Verification items for the finished model (mm, model axes). A direction names the side the tool comes from. Round coordinates to 2 decimals unless told otherwise and drop trailing zeros. Write each loop counter-clockwise with the first axis right and the second up, starting at its lowest first coordinate (ties: lowest second). Pieces come first, ordered by that corner, then holes. Notation, with made-up numbers: (-1.75, -39) -> (57.25, -39) arc R23 cw to (57.25, -15) -> close; hole circle Ø11 at (-24, 6). An arc over 180 degrees is marked (long way). Use CSV: the item, a comma, the result in double quotes.
```python
from build123d import *
from build123d.topology import SkipClean

# Parameters (mm, degrees)
BOSS_EXTRUDE2_DEPTH       = 12.065
BOSS_EXTRUDE3_START       = -15.875
BOSS_EXTRUDE3_OUTLINE_R   = 38.1
BOSS_EXTRUDE3_OUTLINE_R_2 = 25.4
BOSS_EXTRUDE3_DEPTH       = 31.75
SKETCH3_R                 = 9.525
BOSS_EXTRUDE4_DEPTH       = 25.4
SKETCH5_R                 = 4.76
CUT_EXTRUDE1_DEPTH        = 32.4


# Read off the part's stored shape, not the designer's step: Boss-Extrude3
with BuildPart() as part:
    # Sketch1 → Boss-Extrude2 (new, symmetric)
    with SkipClean():  # the faces are left unmerged after this step: merging them gives an invalid solid
        with BuildSketch(Plane(origin=(0, 0, 0), x_dir=(0, 0, -1), z_dir=(1, 0, 0))):
            with BuildLine():
                ThreePointArc((-43.204432116, 19.05), (-114.3, 0), (-43.204432116, -19.05))
                Line((-43.204432116, -19.05), (-59.399479175, -19.05))
                ThreePointArc((-59.399479175, -19.05), (-101.6, 0), (-59.399479175, 19.05))
                Line((-59.399479175, 19.05), (-43.204432116, 19.05))
            make_face()
            with BuildLine():
                Line((-59.399479175, -19.05), (-43.204432116, -19.05))
                ThreePointArc((-43.204432116, -19.05), (-39.398226018, -9.861005618), (-38.1, 0))
                ThreePointArc((-38.1, 0), (-39.398226018, 9.861005618), (-43.204432116, 19.05))
                Line((-43.204432116, 19.05), (-59.399479175, 19.05))
                ThreePointArc((-59.399479175, 19.05), (-53.049479175, 10.450520825), (-50.8, 0))
                ThreePointArc((-50.8, 0), (-53.049479175, -10.450520825), (-59.399479175, -19.05))
            make_face()
            with BuildLine():
                Line((-43.204432116, -19.05), (29.107139607, -19.05))
                ThreePointArc((29.107139607, -19.05), (25.4, 0), (29.107139607, 19.05))
                Line((29.107139607, 19.05), (-43.204432116, 19.05))
                ThreePointArc((-43.204432116, 19.05), (-39.398226018, 9.861005618), (-38.1, 0))
                ThreePointArc((-38.1, 0), (-39.398226018, -9.861005618), (-43.204432116, -19.05))
            make_face()
            with BuildLine():
                Line((29.107139607, -19.05), (43.204432116, -19.05))
                ThreePointArc((43.204432116, -19.05), (38.1, 0), (43.204432116, 19.05))
                Line((43.204432116, 19.05), (29.107139607, 19.05))
                ThreePointArc((29.107139607, 19.05), (25.4, 0), (29.107139607, -19.05))
            make_face()
            with BuildLine():
                Line((29.107139607, 19.05), (43.204432116, 19.05))
                ThreePointArc((43.204432116, 19.05), (57.15, 32.995567884), (76.2, 38.1))
                Line((76.2, 38.1), (76.2, 50.8))
                ThreePointArc((76.2, 50.8), (47.801936686, 42.121134838), (29.107139607, 19.05))
            make_face()
            with BuildLine():
                ThreePointArc((76.2, -38.1), (57.15, -32.995567884), (43.204432116, -19.05))
                Line((43.204432116, -19.05), (29.107139607, -19.05))
                ThreePointArc((29.107139607, -19.05), (47.801936686, -42.121134838), (76.2, -50.8))
                Line((76.2, -50.8), (76.2, -38.1))
            make_face()
        extrude(amount=BOSS_EXTRUDE2_DEPTH, both=True)

    # Boss-Extrude3 outline → Boss-Extrude3 (add)
    with SkipClean():  # the faces are left unmerged after this step: merging them gives an invalid solid
        with BuildSketch(Plane(origin=(0, 0, 0), x_dir=(0, 0, -1), z_dir=(1, 0, 0)).offset(BOSS_EXTRUDE3_START)):
            with Locations((-76.2, 0)):
                Circle(BOSS_EXTRUDE3_OUTLINE_R)
            with Locations((-76.2, 0)):
                Circle(BOSS_EXTRUDE3_OUTLINE_R_2, mode=Mode.SUBTRACT)
        extrude(amount=BOSS_EXTRUDE3_DEPTH)
    add(part.part.scale(1), mode=Mode.REPLACE)  # the faces are merged on a copy

    # Sketch3 → Boss-Extrude4 (add)
    with BuildSketch(Plane(origin=(0, 0, -76.2), x_dir=(-1, 0, 0), z_dir=(0, 0, -1))):
        with Locations((0, -50.8)):
            Circle(SKETCH3_R)
    boss_extrude4 = extrude(amount=-BOSS_EXTRUDE4_DEPTH)

    # Sketch5 → Cut-Extrude1 (cut)
    with BuildSketch(Plane(origin=(0, 0, -76.2), x_dir=(-1, 0, 0), z_dir=(0, 0, -1))):
        with Locations((0, -50.8)):
            Circle(SKETCH5_R)
    cut_extrude1 = extrude(amount=-CUT_EXTRUDE1_DEPTH, mode=Mode.SUBTRACT)

    # Mirror2: Boss-Extrude4, Cut-Extrude1 across plane
    add(boss_extrude4.mirror(Plane.ZX))
    add(cut_extrude1.mirror(Plane.ZX), mode=Mode.SUBTRACT)


solid = part.part
```
Q1. Section check D-D (y = 22). Record the cut outline in (x, z) (3 decimals).
Filled in:
outline,"(-15.875, 45.094) -> (15.875, 45.094) -> (15.875, 63.505) -> (-15.875, 63.505) -> close; (-15.875, 88.895) -> (15.875, 88.895) -> (15.875, 107.306) -> (-15.875, 107.306) -> close; (-12.065, -45.094) -> (12.065, -45.094) -> (12.065, -30.411) -> (-12.065, -30.411) -> close"
Q2. Mould release check, pull along Z, two halves, no side actions. Record for faces 4 (the flat face through (0, -44, -76.2)), 5 (the flat face through (-15.875, -25, 68)), 6 (the cylindrical face through (0.169, -37.742, -42.197)): released by +Z, released by -Z, zero draft, split by the parting line, or undercut.
Filled in:
face 4,"released by -Z"
face 5,"zero draft"
face 6,"undercut"
Q3. Section check B-B (z = 86.5). Record the cut outline in (x, y) (3 decimals), plus the area to 3 significant figures.
Filled in:
outline,"(-15.875, -36.681) -> (15.875, -36.681) -> (15.875, -23.218) -> (-15.875, -23.218) -> close; (-15.875, 23.218) -> (15.875, 23.218) -> (15.875, 36.681) -> (-15.875, 36.681) -> close"
area,"855 mm²"
Q4. Access from +Z, -Z, +X, -X, +Y, -Y to the whole of each face (thin tool, end or side, straight path). Record for faces 1 (the flat face through (0, -56, -50.8)), 2 (the flat face through (0, 19.05, 7)), 3 (the flat face through (0, 56, -50.8)).
Filled in:
face 1,"+Z, +X, -X, -Y"
face 2,"+X, -X, +Y"
face 3,"+Z, +X, -X, +Y"
Q5. Section check A-A (x = 0). Record the cut outline in (y, z) (3 decimals), plus the area to 3 significant figures.
Filled in:
outline,"(-60.325, -76.2) -> (-55.56, -76.2) -> (-55.56, -50.8) -> (-60.325, -50.8) -> close; (-46.04, -76.2) -> (-38.1, -76.2) arc R38.1 cw to (38.1, -76.2) -> (46.04, -76.2) -> (46.04, -50.8) -> (43.994, -50.8) arc R50.8 ccw to (19.05, -29.107) -> (19.05, 43.204) arc R38.1 ccw (long way) to (-19.05, 43.204) -> (-19.05, -29.107) arc R50.8 ccw to (-43.994, -50.8) -> (-46.04, -50.8) -> close; (55.56, -76.2) -> (60.325, -76.2) -> (60.325, -50.8) -> (55.56, -50.8) -> close; hole circle Ø50.8 at (0, 76.2)"
area,"6,950 mm²"
Q6. Section check C-C (y = -4.5). Record the cut outline in (x, z) (3 decimals), plus the area to 3 significant figures.
Filled in:
outline,"(-15.875, 38.367) -> (-12.065, 38.367) -> (-12.065, -38.367) -> (12.065, -38.367) -> (12.065, 38.367) -> (15.875, 38.367) -> (15.875, 51.202) -> (-15.875, 51.202) -> close; (-15.875, 101.198) -> (15.875, 101.198) -> (15.875, 114.033) -> (-15.875, 114.033) -> close"
area,"2,670 mm²"
Q7. Material ranges on L1, parallel to Y at x = 0, z = -60.25 (3 decimals); L2, parallel to Y at x = 0, z = -68 (3 decimals); L3, parallel to Y at x = -13.65, z = 76.2, recorded low to high.
Filled in:
L1,"-60.325 to -55.56, -46.04 to -34.601, 34.601 to 46.04, 55.56 to 60.325"
L2,"-60.325 to -55.56, -46.04 to -37.207, 37.207 to 46.04, 55.56 to 60.325"
L3,"-38.1 to -25.4, 25.4 to 38.1"
Q8. Go/stop test with flat-tipped pins: P1, Ø8, axis at x = -4.5, y = -52, coming from the +Z side; P2, Ø12, axis at x = 0, z = -4, coming from the +Y side; P3, Ø8, axis at y = -22.5, z = -36, coming from the +X side (3 decimals). Record where each tip stops, or that it passes through.
Filled in:
P1,"z = -50.8"
P2,"y = 19.05"
P3,"x = 12.065"
